Part model, mm, in its own coordinate system. Face numbers are marked on the shaded views. Coordinates: 2 decimals unless noted, no trailing zeros. Write each loop counter-clockwise with the first axis right and the second up, starting at its lowest first coordinate (ties: lowest second). Pieces come first, ordered by that corner, then holes. Notation, with made-up numbers: (41.5, 1.5) -> (100.5, 1.5) arc R11 cw to (100.5, 11.5) -> close; hole circle Ø2 at (25.25, 63.25). An arc over 180 degrees is marked (long way). Write item = value, one per line.
from build123d import *

# Parameters (mm, degrees)
SKETCH1_R           = 12.5
SKETCH1_R_2         = 10.5
BOSS_EXTRUDE1_DEPTH = 45
SKETCH3_W           = 2.4
SKETCH3_H           = 23.000586798
BOSS_EXTRUDE3_DEPTH = 45
SKETCH4_R           = 3.019619096
BOSS_EXTRUDE4_DEPTH = 45
SKETCH5_R           = 2
CUT_EXTRUDE1_DEPTH  = 49.347699015


with BuildPart() as part:
    # Sketch1 → Boss-Extrude1 (new body)
    with BuildSketch(Plane(origin=(0, 0, 0), x_dir=(1, 0, 0), z_dir=(0, 1, 0))):
        with Locations(Location((0, 0, 0), (0, 0, 90))):
            Circle(SKETCH1_R)
        with Locations(Location((0, 0, 0), (0, 0, 90))):
            Circle(SKETCH1_R_2, mode=Mode.SUBTRACT)
    extrude(amount=BOSS_EXTRUDE1_DEPTH)

    # Sketch3 → Boss-Extrude3 (add, through all)
    with BuildSketch(Plane(origin=(0, 45, 0), x_dir=(1, 0, 0), z_dir=(0, 1, 0))):
        with Locations((0, 0.0942647)):
            Rectangle(SKETCH3_W, SKETCH3_H)
    extrude(amount=-BOSS_EXTRUDE3_DEPTH)

    # Sketch4 → Boss-Extrude4 (add, through all)
    with BuildSketch(Plane(origin=(0, 45, 0), x_dir=(1, 0, 0), z_dir=(0, 1, 0))):
        with Locations((0, 6.928455449)):
            Circle(SKETCH4_R)
    extrude(amount=-BOSS_EXTRUDE4_DEPTH)

    # Sketch5 → Cut-Extrude1 (cut, through all)
    with BuildSketch(Plane(origin=(0, 45, 0), x_dir=(1, 0, 0), z_dir=(0, 1, 0))):
        with Locations(Location((0, 6.928455449, 0), (0, 0, 270))):
            Circle(SKETCH5_R)
    extrude(amount=-CUT_EXTRUDE1_DEPTH, mode=Mode.SUBTRACT)


solid = part.part
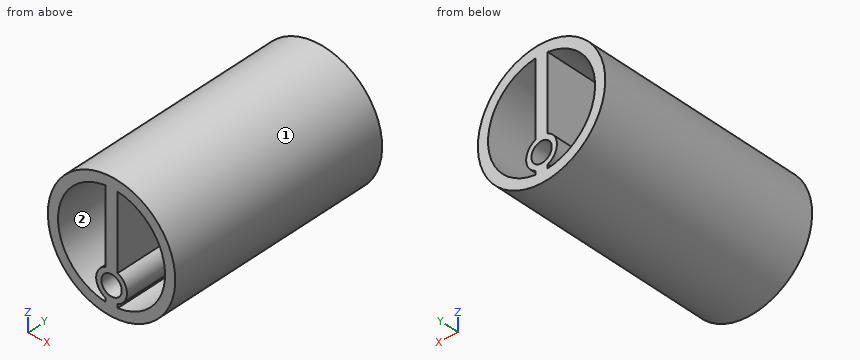
Q1. Saw through at A-A on x = 0. Give the cut face in (y, z).
Model answer:
outline = (0, -12.5) -> (45, -12.5) -> (45, -8.93) -> (0, -8.93) -> close; (0, -4.93) -> (45, -4.93) -> (45, 12.5) -> (0, 12.5) -> close
Q2. Saw through at B-B on z = 0. Give the cut face in (x, y), and give its area (3 significant figures).
Model answer:
outline = (-12.5, 0) -> (-10.5, 0) -> (-10.5, 45) -> (-12.5, 45) -> close; (-1.2, 0) -> (1.2, 0) -> (1.2, 45) -> (-1.2, 45) -> close; (10.5, 0) -> (12.5, 0) -> (12.5, 45) -> (10.5, 45) -> close
area = 288 mm²
Q3. Probe line 1 (X direction, y = 24, z = 7.5); line 2 (X direction, y = 34.5, z = -9.5); line 3 (Z direction, x = 1.75, y = 27.5). List the from-to ranges inside material, lowest first. Write a range as from..to.
Model answer:
line_1 = -10..-7.35, -1.2..1.2, 7.35..10
line_2 = -8.12..-4.47, -1.58..1.58, 4.47..8.12
line_3 = -12.38..-10.35, -9.39..-7.9, -5.96..-4.47, 10.35..12.38
Q4. Pin check, flat tips, straight feed: pin 1 (6.5 mm diameter, centred on x = 0, z = -6.93, fed in from +Y); pin 2 (0.8 mm diameter, centred on y = 33, z = -10, fed in from -X); pin 3 (12 mm diameter, centred on x = 7.5, y = 24.5, fed in from -Z); pin 4 (4.5 mm diameter, centred on y = 28.5, z = 5.5, fed in from -X). Stop position of each tip, or through.
Model answer:
pin_1 = 45
pin_2 = -8.01
pin_3 = -12.41
pin_4 = -12.07
Q5. Saw through at C-C on y = 24. Give the cut face in (x, z).
Model answer:
outline = circle Ø25 at (0, 0); hole circle Ø4 at (0, -6.93); hole (-1.2, -10.43) -> (-1.2, -9.7) arc R3.02 cw to (-1.2, -4.16) -> (-1.2, 10.43) arc R10.5 ccw to start; hole (1.2, -10.43) arc R10.5 ccw to (1.2, 10.43) -> (1.2, -4.16) arc R3.02 cw to (1.2, -9.7) -> close
Q6. Saw through at D-D on z = -3. Give the cut face in (x, y).
Model answer:
outline = (-12.13, 0) -> (-10.06, 0) -> (-10.06, 45) -> (-12.13, 45) -> close; (-1.2, 0) -> (1.2, 0) -> (1.2, 45) -> (-1.2, 45) -> close; (10.06, 0) -> (12.13, 0) -> (12.13, 45) -> (10.06, 45) -> close
Q7. Mould opens along X. For the marked faces 1 and 2 say: released by +X, released by -X, zero draft, split by the parting line, or undercut.
Model answer:
face_1 = split by the parting line
face_2 = undercut
